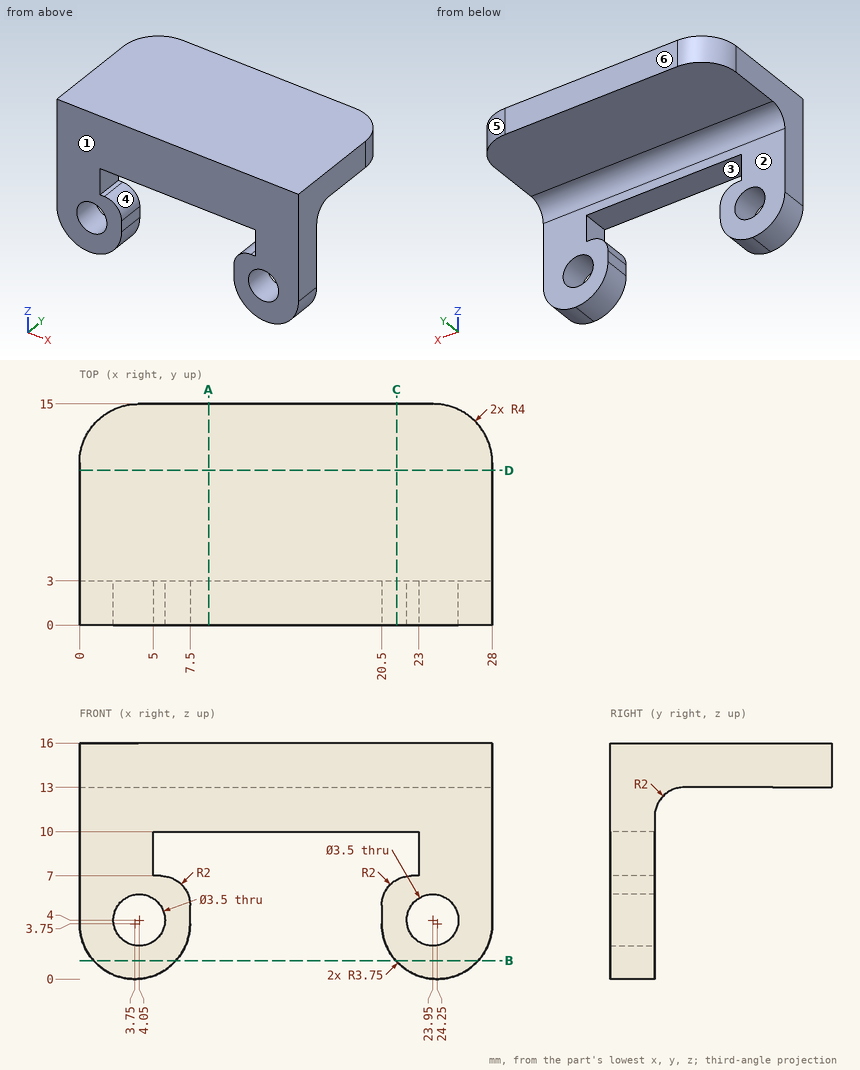
Check sheet for the drawn part. Datum: minimum x, y, z corner. Units: mm. A direction names the side the tool comes from. Give positions to 0.01 mm unless a question says otherwise; leave off trailing zeros. Order: outer loops, then holes, each group sorted by start corner. A loop starts at its lowest first (then second) coordinate and runs counter-clockwise, first axis right, second up. Notation, with made-up numbers: (22, -13.5) - (70, -13.5) arc R5 cw to (70, -6.5) - close; hole circle Ø7 at (16, -26). An arc over 180 degrees is marked (long way). Write item = value, one per line. Start each with the question number.
1) Access from +Z, -Z, +X, -X, +Y, -Y to the whole of each face (thin tool, end or side, straight path). Record for the marked faces 1, 2 and 3.
2) Section check D-D (y = 10.5). Enter the section's corners in (x, z), then the cut area to 3 significant figures.
3) Section check A-A (x = 8.75). Enter the section's corners in (y, z).
4) Scan lines: L1, parallel to X at y = 1.65, z = 4; L2, parallel to Y at x = 3, z = 6.75; L3, parallel to X at y = 2, z = 2.5. Record each from-to range of solid material in increasing order.
5) Gauge pin test, flat ends, axial feed: pin 1 Ø4 at (x, y) = (19, 2) entering from -Z; pin 2 Ø9 at (x, z) = (16.5, 3.5) entering from +Y; pin 3 Ø3.5 at (x, y) = (9.5, 1.5) entering from -Z. Record the tip position at first contact, or that the pin passes through.
6) Draft check along X on the marked faces 4, 5 and 6. Enter one of: released by +X, released by -X, zero draft, split by the parting line, or undercut.
7) Section check B-B (z = 1.25). Enter the section's corners in (x, y), then the cut area to 3 significant figures.
8) Section check C-C (x = 21.5). Enter the section's corners in (y, z), then the cut area to 3 significant figures.
Geometry check:
q1.face_1 = +Z, -Z, +X, -X, -Y
q1.face_2 = -Z, +X, -X, +Y
q1.face_3 = +Y, -Y
q2.outline = (0, 13) - (28, 13) - (28, 16) - (0, 16) - close
q2.area = 84.0 mm2
q3.outline = (0, 10) - (3, 10) - (3, 11) arc R2 cw to (5, 13) - (15, 13) - (15, 16) - (0, 16) - close
q4.L1 = 0 to 2.3, 5.8 to 7.5, 20.5 to 22.2, 25.7 to 28
q4.L2 = 0 to 3
q4.L3 = 0.21 to 3.15, 4.95 to 7.29, 20.71 to 23.05, 24.85 to 27.79
q5.pin_1 = 1.88
q5.pin_2 = 3
q5.pin_3 = 10
q6.face_4 = undercut
q6.face_5 = released by +X
q6.face_6 = zero draft
q7.outline = (0.95, 0) - (6.55, 0) - (6.55, 3) - (0.95, 3) - close; (21.45, 0) - (27.05, 0) - (27.05, 3) - (21.45, 3) - close
q7.area = 33.5 mm2
q8.outline = (0, 1.2) - (3, 1.2) - (3, 6.73) - (0, 6.73) - close; (0, 10) - (3, 10) - (3, 11) arc R2 cw to (5, 13) - (15, 13) - (15, 16) - (0, 16) - close
q8.area = 71.5 mm2
